```python
from build123d import *

# Parameters (mm, degrees)
F0_R     = 1.75
F1_DEPTH = 4
F2_DEPTH = 15
F3_R     = 5
F4_R     = 1


# Not quite as in the source:
# - a feature names something its author has since deleted; it is built from what else it names


with BuildPart() as f1:
    # F0 (on Top) → F1 (new body)
    with BuildSketch(Plane.XY):
        with BuildLine():
            Line((-33.9130103109, 52.4991212465), (-41.2382205381, 63.8389314357))
            ThreePointArc((-41.2382205381, 63.8389314357), (-44.9500240756, 61.2820963709), (-48.5037329382, 58.5097247563))
            ThreePointArc((-48.5037329382, 58.5097247563), (-49.20563764, 57.9206804556), (-49.9003894351, 57.3232163633))
            ThreePointArc((-49.9003894351, 57.3232163633), (-44.1059919264, 55.4322284704), (-41.6292667465, 49.8629637))
            ThreePointArc((-41.6292667465, 49.8629637), (-42.2108537269, 46.9671803363), (-43.8654164238, 44.5205036131))
            ThreePointArc((-43.8654164238, 44.5205036131), (-39.0932922784, 48.7643773551), (-33.9130103109, 52.4991212465))
        make_face()
        with Locations((-40.8724684836, 56.828173647)):
            Circle(F0_R, mode=Mode.SUBTRACT)
        with BuildLine():
            ThreePointArc((-49.4610434567, 59.6645219554), (-51.9749220296, 57.4878898553), (-54.3931164452, 55.2054244018))
            ThreePointArc((-54.3931164452, 55.2054244018), (-52.3271541158, 56.6470271117), (-49.9003894351, 57.3232163633))
            ThreePointArc((-49.9003894351, 57.3232163633), (-49.20563764, 57.9206804556), (-48.5037329382, 58.5097247563))
            Line((-48.5037329382, 58.5097247563), (-49.4610434568, 59.6645219554))
        make_face()
        with BuildLine():
            Line((-69.4199358602, 39.5800459158), (-67.3257807989, 38.3860552782))
            ThreePointArc((-67.3257807989, 38.3860552782), (-61.4377349925, 47.2403928751), (-54.3931164452, 55.2054244018))
            ThreePointArc((-54.3931164452, 55.2054244018), (-51.9749220296, 57.4878898553), (-49.4610434567, 59.6645219554))
            Line((-49.4610434568, 59.6645219554), (-50.9995194055, 61.5203750796))
            ThreePointArc((-50.9995194055, 61.5203750796), (-61.2009461738, 51.382406687), (-69.4199358602, 39.5800459158))
        make_face()
        with BuildLine():
            ThreePointArc((-49.4610434567, 59.6645219554), (-45.8371956034, 62.4916114308), (-42.0521327855, 65.0989103456))
            Line((-42.0521327855, 65.0989103456), (-43.360156037, 67.123799043))
            ThreePointArc((-43.360156037, 67.123799043), (-47.2629524833, 64.4354006125), (-50.9995194055, 61.5203750796))
            Line((-50.9995194055, 61.5203750796), (-49.4610434568, 59.6645219554))
        make_face()
        with BuildLine():
            Line((-41.2382205381, 63.8389314357), (-42.0521327855, 65.0989103456))
            ThreePointArc((-42.0521327855, 65.0989103456), (-45.8371956034, 62.4916114308), (-49.4610434567, 59.6645219554))
            Line((-49.4610434568, 59.6645219554), (-48.5037329382, 58.5097247563))
            ThreePointArc((-48.5037329382, 58.5097247563), (-44.9500240756, 61.2820963709), (-41.2382205381, 63.8389314357))
        make_face()
        with BuildLine():
            ThreePointArc((-54.3931164452, 55.2054244018), (-61.4377349925, 47.2403928751), (-67.3257807989, 38.3860552782))
            Line((-67.3257807989, 38.3860552782), (-66.0227011705, 37.6430993696))
            ThreePointArc((-66.0227011705, 37.6430993696), (-61.6490099795, 44.4454673566), (-56.577269857, 50.7445813415))
            ThreePointArc((-56.577269857, 50.7445813415), (-55.8651839567, 53.1610569882), (-54.3931164452, 55.2054244018))
        make_face()
        with BuildLine():
            ThreePointArc((-49.9003894351, 57.3232163633), (-52.3271541158, 56.6470271117), (-54.3931164452, 55.2054244018))
            ThreePointArc((-54.3931164452, 55.2054244018), (-55.8651839567, 53.1610569882), (-56.577269857, 50.7445813415))
            ThreePointArc((-56.577269857, 50.7445813415), (-55.8760464089, 51.5157008854), (-55.1643138946, 52.277131449))
            ThreePointArc((-55.1643138946, 52.277131449), (-53.6912700872, 54.4930960436), (-51.453714731, 55.9331318663))
            ThreePointArc((-51.453714731, 55.9331318663), (-50.6818181556, 56.6334998781), (-49.9003894351, 57.3232163633))
        make_face()
        with BuildLine():
            ThreePointArc((-41.6292667465, 49.8629637), (-44.1059919264, 55.4322284704), (-49.9003894351, 57.3232163633))
            ThreePointArc((-49.9003894351, 57.3232163633), (-50.6818181556, 56.6334998781), (-51.453714731, 55.9331318663))
            ThreePointArc((-51.453714731, 55.9331318663), (-45.4454448113, 55.2182840406), (-42.6292667465, 49.8629637))
            ThreePointArc((-42.6292667465, 49.8629637), (-50.3585335071, 43.4802602578), (-55.1643138946, 52.277131449))
            ThreePointArc((-55.1643138946, 52.277131449), (-55.8760464089, 51.5157008854), (-56.577269857, 50.7445813415))
            ThreePointArc((-56.577269857, 50.7445813415), (-52.4273596413, 43.1270462972), (-43.8654164238, 44.5205036131))
            ThreePointArc((-43.8654164238, 44.5205036131), (-42.2108537269, 46.9671803363), (-41.6292667465, 49.8629637))
        make_face()
        with BuildLine():
            ThreePointArc((-56.577269857, 50.7445813415), (-61.6490099795, 44.4454673566), (-66.0227011705, 37.6430993696))
            Line((-66.0227011705, 37.6430993696), (-54.2949845152, 30.9564961921))
            ThreePointArc((-54.2949845152, 30.9564961921), (-49.5465604503, 38.0970910641), (-43.8654164238, 44.5205036131))
            ThreePointArc((-43.8654164238, 44.5205036131), (-52.4273596413, 43.1270462972), (-56.577269857, 50.7445813415))
        make_face()
        with Locations((-58.1049998349, 39.0359961341)):
            Circle(F0_R, mode=Mode.SUBTRACT)
        with BuildLine():
            ThreePointArc((-43.8654164238, 44.5205036131), (-49.5465604503, 38.0970910641), (-54.2949845152, 30.9564961921))
            Line((-54.2949845152, 30.9564961921), (-51.8884792508, 29.5844178737))
            ThreePointArc((-51.8884792508, 29.5844178737), (-43.387995367, 41.0503826769), (-32.4098910344, 50.1722136548))
            Line((-32.4098910344, 50.1722136548), (-33.9130103109, 52.4991212465))
            ThreePointArc((-33.9130103109, 52.4991212465), (-39.0932922784, 48.7643773551), (-43.8654164238, 44.5205036131))
        make_face()
    extrude(amount=-F1_DEPTH)

    # F0 (on Top) → F2 (join)
    with BuildSketch(Plane.XY):
        with BuildLine():
            ThreePointArc((-49.9003894351, 57.3232163633), (-52.3271541158, 56.6470271117), (-54.3931164452, 55.2054244018))
            ThreePointArc((-54.3931164452, 55.2054244018), (-55.8651839567, 53.1610569882), (-56.577269857, 50.7445813415))
            ThreePointArc((-56.577269857, 50.7445813415), (-55.8760464089, 51.5157008854), (-55.1643138946, 52.277131449))
            ThreePointArc((-55.1643138946, 52.277131449), (-53.6912700872, 54.4930960436), (-51.453714731, 55.9331318663))
            ThreePointArc((-51.453714731, 55.9331318663), (-50.6818181556, 56.6334998781), (-49.9003894351, 57.3232163633))
        make_face()
        with BuildLine():
            ThreePointArc((-41.6292667465, 49.8629637), (-44.1059919264, 55.4322284704), (-49.9003894351, 57.3232163633))
            ThreePointArc((-49.9003894351, 57.3232163633), (-50.6818181556, 56.6334998781), (-51.453714731, 55.9331318663))
            ThreePointArc((-51.453714731, 55.9331318663), (-45.4454448113, 55.2182840406), (-42.6292667465, 49.8629637))
            ThreePointArc((-42.6292667465, 49.8629637), (-50.3585335071, 43.4802602578), (-55.1643138946, 52.277131449))
            ThreePointArc((-55.1643138946, 52.277131449), (-55.8760464089, 51.5157008854), (-56.577269857, 50.7445813415))
            ThreePointArc((-56.577269857, 50.7445813415), (-52.4273596413, 43.1270462972), (-43.8654164238, 44.5205036131))
            ThreePointArc((-43.8654164238, 44.5205036131), (-42.2108537269, 46.9671803363), (-41.6292667465, 49.8629637))
        make_face()
    extrude(amount=-F2_DEPTH)

    # F3
    f3_edges = [f1.edges().sort_by_distance(p)[0] for p in [
        (-43.360156, 67.123799, -2),
        (-32.409891, 50.172214, -2),
        (-69.419936, 39.580046, -2),
        (-51.888479, 29.584418, -2),
    ]]
    fillet(f3_edges, radius=F3_R)

    # F4
    f4_edges = [f1.edges().sort_by_distance(p)[0] for p in [
        (-43.865417, 44.520503, -4),
        (-46.804819, 43.792796, 0),
    ]]
    fillet(f4_edges, radius=F4_R)


solid = f1.part
```
Verification items for the finished model (mm, model axes). Give positions to 0.01 mm unless a question says otherwise; leave off trailing zeros. Write each loop counter-clockwise with the first axis right and the second up, starting at its lowest first coordinate (ties: lowest second). Pieces come first, ordered by that corner, then holes. Notation, with made-up numbers: M -35.5,-17 L -6.5,-17 A11 ccw -6.5,0 Z; hole C 46.5,20 d7. An arc over 180 degrees is marked long. One line per question, with ' | ' between items.
1) Mould release check, pull along Y, two halves, no side actions. Record for faces 1 (the flat face through (-51, 41, -4)), 2 (the cylindrical face through (-43.481, 40.952, -1.972)), 3 (the cylindrical face through (-57.3, 37.48, -1.97)), 4 (the cylindrical face through (-50.18, 43.45, -7.9)): released by +Y, released by -Y, zero draft, split by the parting line, or undercut.
Result:
face 1: zero draft | face 2: released by -Y | face 3: undercut | face 4: undercut
2) Gauge pin test, flat ends, axial feed: pin 1 Ø5 at (x, y) = (-62, 39) entering from -Z; pin 2 Ø1 at (y, z) = (53.5, -9) entering from -X; pin 3 Ø5 at (x, z) = (-44, -8.5) entering from +Y. Record the tip position at first contact, or that the pin passes through.
Result:
pin 1: stops at z = -4 | pin 2: stops at x = -55.94 | pin 3: stops at y = 56.89
3) Section check D-D on y = 36. Enter the section's corners in (x, z).
Result:
outline: M -63.14,-4 L -47.66,-4 L -47.66,0 L -63.14,0 Z
4) Section check B-B on x = -37. Enter the section's corners in (y, z), plus the area to 3 significant figures.
Result:
outline: M 46.89,-4 L 57.28,-4 L 57.28,0 L 46.89,0 Z | area: 41.6 mm2
5) Section check A-A on z = -7.25. Enter the section's corners in (x, y).
Result:
outline: C -49.13,49.86 d15; hole C -49.13,49.86 d13
6) Thickness scan on line 1 along Z through (x, y) = (-41.5, 44); line 2 along Y through (x, z) = (-42, -1); line 3 along Y through (x, z) = (-48.5, -10.25). Record the ranges inside material, lowest first. Write a range as [from, to].
Result:
line 1: z = [-4, 0] | line 2: y = [42.47, 55.49], [58.17, 64.24] | line 3: y = [42.39, 43.39], [56.33, 57.34]
7) Section check C-C on z = -2. State how many separate pieces and enclosed holes the cut face has, plus the area to 3 significant figures.
Result:
separate pieces: 1 | enclosed holes: 3 | area: 502 mm2
